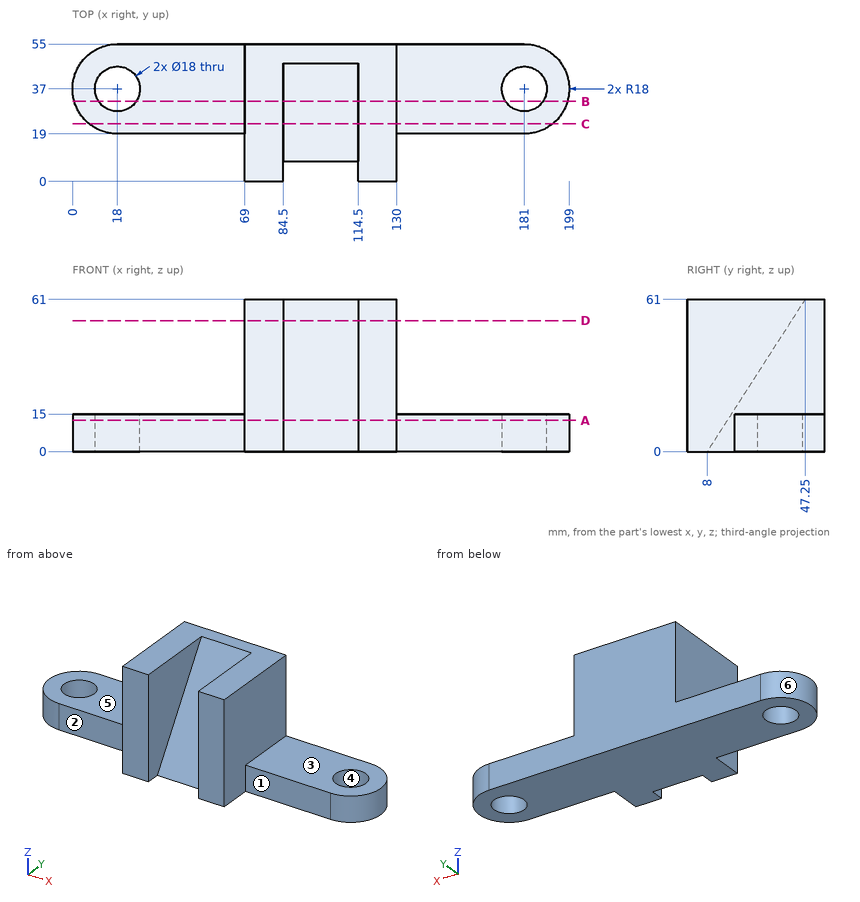
The drawing under review shows one solid part. Ordinate dimensions are in mm from its lowest x, y, z. A direction names the side the tool comes from. Coordinates: 2 decimals unless noted, no trailing zeros. Write each loop counter-clockwise with the first axis right and the second up, starting at its lowest first coordinate (ties: lowest second). Pieces come first, ordered by that corner, then holes. Notation, with made-up numbers: (3.25, 56) -> (43.25, 56) arc R19 cw to (43.25, 63) -> close; hole circle Ø7 at (88.25, 25.25). An arc over 180 degrees is marked (long way). Write each question's results on one line, items separated by ' | '. Start each with the question number.
1) Consider section C-C (y = 23). Write out the cut boundary in (x, z), plus the area to 3 significant figures.
2) Wall thickness on L1, parallel to X at y = 37, z = 6.5; L2, parallel to Y at x = 18, z = 4.5; L3, parallel to X at y = 17, z = 46: over which ranges is each line inside the solid? List them lowest first. Write a range as [from, to].
3) Consider section B-B (y = 32). Write out the cut boundary in (x, z), plus the area to 3 significant figures.
4) For the marked faces 1, 2 and 3, list the 3-axis set-ups (+Z, -Z, +X, -X, +Y, -Y) from which the entire face can be reached by the end or side of a thin tool; tool diameter is ignored.
5) The part is to be moulded in two halves that separate along X. For the marked faces 4, 5 and 6, say which applies: +X half, -X half, draft (parallel to the pull), parting line (faces both ways), or undercut.
6) Insertion check: pin 1 (6 mm diameter, centred on x = 92.5, y = 33.5, fed in from +Z); pin 2 (12 mm diameter, centred on x = 44.5, z = 7.5, fed in from -Y); pin 3 (1.5 mm diameter, centred on y = 33, z = 9.5, fed in from +X). Each pin has a flat end and moves straight along its axis. Give the tip position at first contact, or say it passes through.
7) Consider section D-D (z = 52.5). Write out the cut boundary in (x, y).
8) Consider section A-A (z = 12.5). Write out the cut boundary in (x, y).
Geometry says:
1) outline: (6.69, 0) -> (192.31, 0) -> (192.31, 15) -> (130, 15) -> (130, 61) -> (114.5, 61) -> (114.5, 23.31) -> (84.5, 23.31) -> (84.5, 61) -> (69, 61) -> (69, 15) -> (6.69, 15) -> close | area: 4,460 mm^2
2) L1: [0, 9], [27, 172], [190, 199] | L2: [19, 28], [46, 55] | L3: [69, 84.5], [114.5, 130]
3) outline: (0.71, 0) -> (10.52, 0) -> (10.52, 15) -> (0.71, 15) -> close; (25.48, 0) -> (173.52, 0) -> (173.52, 15) -> (130, 15) -> (130, 61) -> (114.5, 61) -> (114.5, 37.3) -> (84.5, 37.3) -> (84.5, 61) -> (69, 61) -> (69, 15) -> (25.48, 15) -> close; (188.48, 0) -> (198.29, 0) -> (198.29, 15) -> (188.48, 15) -> close | area: 4,610 mm^2
4) face 1: +Z, -Z, +X, -Y | face 2: +Z, -Z, -X, -Y | face 3: +Z, +X, +Y, -Y
5) face 4: undercut | face 5: draft | face 6: -X half
6) pin 1: z = 44.29 | pin 2: y = 19 | pin 3: x = 198.7
7) outline: (69, 0) -> (84.5, 0) -> (84.5, 41.78) -> (114.5, 41.78) -> (114.5, 0) -> (130, 0) -> (130, 55) -> (69, 55) -> close
8) outline: (18, 19) -> (69, 19) -> (69, 0) -> (84.5, 0) -> (84.5, 16.04) -> (114.5, 16.04) -> (114.5, 0) -> (130, 0) -> (130, 19) -> (181, 19) arc R18 ccw to (181, 55) -> (18, 55) arc R18 ccw to start; hole circle Ø18 at (18, 37); hole circle Ø18 at (181, 37)
